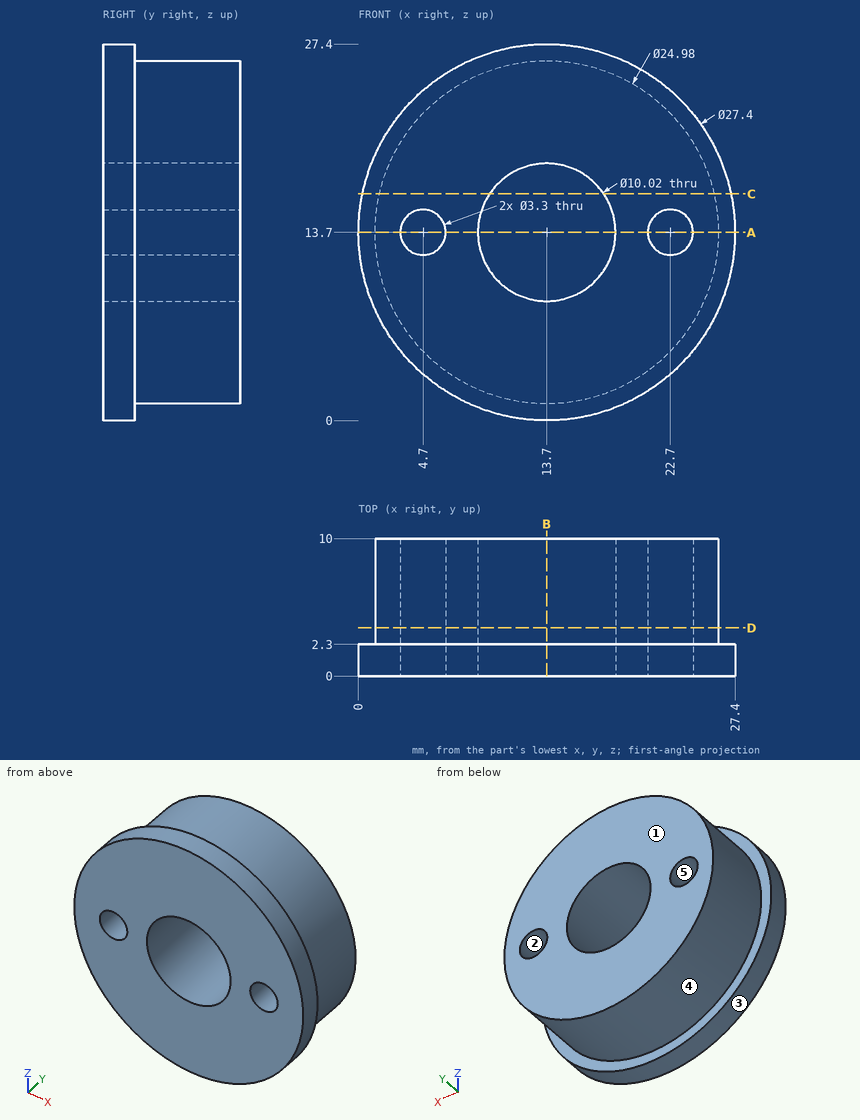
The drawing under review shows one solid part. Ordinate dimensions are in mm from its lowest x, y, z. A direction names the side the tool comes from. Coordinates: 2 decimals unless noted, no trailing zeros. Order: outer loops, then holes, each group sorted by start corner. A loop starts at its lowest first (then second) coordinate and runs counter-clockwise, first axis right, second up. Notation, with made-up numbers: (46, 70) - (89, 70) arc R31 ccw to (89, 102) - close; hole circle Ø8 at (53.5, -30). An arc over 180 degrees is marked (long way). Put each result on its own line as item: value.
1) Tool access review of the marked faces 4 and 5: name each direction out of +Z, -Z, +X, -X, +Y, -Y from which nothing blocks a thin tool from reaching the whole face with its end or side.
Response values:
face 4: +Y
face 5: +Y, -Y
2) Take a section at C-C, the plane z = 16.5. Give the boundary of the cut face in (x, y), and give its area (3 significant figures).
Response values:
outline: (0.29, 0) - (9.55, 0) - (9.55, 10) - (1.53, 10) - (1.53, 2.3) - (0.29, 2.3) - close; (17.85, 0) - (27.11, 0) - (27.11, 2.3) - (25.87, 2.3) - (25.87, 10) - (17.85, 10) - close
area: 166 mm²
3) Insertion check: P1, Ø6, axis at x = 24, y = 5.5, coming from the -Z side; P2, Ø1.5, axis at y = 2, z = 6.5, coming from the +X side; P3, Ø2, axis at x = 24.5, y = 6.5, coming from the -Z side; P4, Ø2, axis at x = 22.7, z = 13.7, coming from the +Y side. Each pin has a flat end and moves straight along its axis. Give the tip position at first contact, or say it passes through.
Response values:
P1: stops at z = 3.57
P2: stops at x = 25.79
P3: stops at z = 5.96
P4: passes through
4) Take a section at A-A, the plane z = 13.7. Give the boundary of the cut face in (x, y), and give its area (3 significant figures).
Response values:
outline: (0, 0) - (3.05, 0) - (3.05, 10) - (1.21, 10) - (1.21, 2.3) - (0, 2.3) - close; (6.35, 0) - (8.69, 0) - (8.69, 10) - (6.35, 10) - close; (18.71, 0) - (21.05, 0) - (21.05, 10) - (18.71, 10) - close; (24.35, 0) - (27.4, 0) - (27.4, 2.3) - (26.19, 2.3) - (26.19, 10) - (24.35, 10) - close
area: 89.2 mm²
5) Take a section at B-B, the plane x = 13.7. Give the boundary of the cut face in (y, z), and give its area (3 significant figures).
Response values:
outline: (0, 0) - (2.3, 0) - (2.3, 1.21) - (10, 1.21) - (10, 8.69) - (0, 8.69) - close; (0, 18.71) - (10, 18.71) - (10, 26.19) - (2.3, 26.19) - (2.3, 27.4) - (0, 27.4) - close
area: 155 mm²
6) Take a section at D-D, the plane y = 3.5. Give the boundary of the cut face in (x, z).
Response values:
outline: circle Ø24.98 at (13.7, 13.7); hole circle Ø3.3 at (4.7, 13.7); hole circle Ø10.02 at (13.7, 13.7); hole circle Ø3.3 at (22.7, 13.7)
7) Wall thickness on L1, parallel to X at y = 6.25, z = 13.7; L2, parallel to X at y = 3.75, z = 11.25; L3, parallel to X at y = 2.5, z = 11.75: over which ranges is each line inside the solid? List them lowest first. Write a range as from..to.
Response values:
L1: x = 1.21..3.05, 6.35..8.69, 18.71..21.05, 24.35..26.19
L2: x = 1.45..9.33, 18.07..25.95
L3: x = 1.36..9.09, 18.31..26.04
8) The part is to be moulded in two halves that separate along X. For the marked faces 1, 2 and 3, say which applies: released by +X, released by -X, zero draft, split by the parting line, or undercut.
Response values:
face 1: zero draft
face 2: undercut
face 3: split by the parting line
